```python
from build123d import *

# Parameters (mm, degrees)
SKETCH1_W          = 6.35
SKETCH1_H          = 6.35
EXTRUDE1_DEPTH     = 7.874
SKETCH2_W          = 1.4478
SKETCH2_H          = 1.4478
EXTRUDE2_DEPTH     = 0.635
SKETCH3_W          = 1.016
SKETCH3_H          = 1.016
EXTRUDE3_DEPTH     = 3.937
SKETCH4_R          = 1.693605641
CUT_EXTRUDE1_DEPTH = 0.254
SKETCH5_R          = 0.4826
EXTRUDE4_DEPTH     = 4.826
SKETCH6_W          = 6.35
SKETCH6_H          = 6.35
EXTRUDE5_DEPTH     = 0.9652
SKETCH7_R          = 1.8542
EXTRUDE6_DEPTH     = 6.1468
SKETCH9_R          = 1.236423773
CUT_EXTRUDE2_DEPTH = 5.658092827
SKETCH10_R         = 0.406972167
EXTRUDE7_DEPTH     = 5.658092827
CHAMFER1_SIZE      = 0.508
CHAMFER1_SIZE2     = 0.126658625


with BuildPart() as part:
    # Sketch1 → Extrude1 (new body)
    with BuildSketch(Plane(origin=(0, 0, 0), x_dir=(1, 0, 0), z_dir=(0, 1, 0))):
        with Locations((3.175, 3.175)):
            Rectangle(SKETCH1_W, SKETCH1_H)
    extrude(amount=EXTRUDE1_DEPTH)

    # Sketch2 → Extrude2 (add)
    with BuildSketch(Plane.XZ):
        with Locations((5.6261, -0.7239)):
            Rectangle(SKETCH2_W, SKETCH2_H)
        with Locations((5.6261, -5.6261)):
            Rectangle(SKETCH2_W, SKETCH2_H)
        with Locations((0.7239, -5.6261)):
            Rectangle(SKETCH2_W, SKETCH2_H)
        with Locations((0.7239, -0.7239)):
            Rectangle(SKETCH2_W, SKETCH2_H)
    extrude(amount=EXTRUDE2_DEPTH)

    # Sketch3 → Extrude3 (add)
    with BuildSketch(Plane.XZ.offset(0.635)):
        with Locations((5.715, -0.617649022)):
            Rectangle(SKETCH3_W, SKETCH3_H)
        with Locations((5.715, -5.697649022)):
            Rectangle(SKETCH3_W, SKETCH3_H)
        with Locations((0.635, -5.697649022)):
            Rectangle(SKETCH3_W, SKETCH3_H)
        with Locations((0.635, -0.617649022)):
            Rectangle(SKETCH3_W, SKETCH3_H)
    extrude(amount=EXTRUDE3_DEPTH)

    # Sketch4 → Cut-Extrude1 (cut)
    with BuildSketch(Plane.XZ):
        with Locations(Location((3.175, -3.175, 0), (0, 0, 270))):
            Circle(SKETCH4_R)
    extrude(amount=-CUT_EXTRUDE1_DEPTH, mode=Mode.SUBTRACT)

    # Sketch5 → Extrude4 (add)
    with BuildSketch(Plane.XZ.offset(-0.254)):
        with Locations(Location((3.175, -3.175, 0), (0, 0, 90))):
            Circle(SKETCH5_R)
    extrude(amount=EXTRUDE4_DEPTH)

    # Sketch6 → Extrude5 (add)
    with BuildSketch(Plane.XY):
        with Locations((3.175, 4.699)):
            Rectangle(SKETCH6_W, SKETCH6_H)
    extrude(amount=EXTRUDE5_DEPTH)

    # Sketch7 → Extrude6 (add)
    with BuildSketch(Plane.XY.offset(0.9652)):
        with Locations((3.175, 4.9022)):
            Circle(SKETCH7_R)
    extrude(amount=EXTRUDE6_DEPTH)

    # Sketch8 → Cut-Revolve1 (revolve, cut)
    with BuildSketch(Plane(origin=(0, 4.9022, 0), x_dir=(-1, 0, 0), z_dir=(0, 1, 0))):
        Polygon((-4.767796954, 7.112), (-5.0292, 6.777141647), (-5.0292, 3.959542683), (-4.884349235, 3.83568961), (-4.884349235, 3.47951039), (-5.0292, 3.363076056), (-5.0292, 0.9652), (-5.650551893, 0.9652), (-5.650551893, 7.801111761), align=None)
    revolve(axis=Axis((3.175, 4.9022, 7.112), (0, 0, -1)), mode=Mode.SUBTRACT)

    # Sketch9 → Cut-Extrude2 (cut)
    with BuildSketch(Plane.XY.offset(7.112)):
        with Locations((3.175, 4.9022)):
            Circle(SKETCH9_R)
    extrude(amount=-CUT_EXTRUDE2_DEPTH, mode=Mode.SUBTRACT)

    # Sketch10 → Extrude7 (add)
    with BuildSketch(Plane.XY.offset(1.453907173)):
        with Locations((3.175, 4.9022)):
            Circle(SKETCH10_R)
    extrude(amount=EXTRUDE7_DEPTH)

    # Chamfer1
    chamfer1_edges = [part.edges().sort_by_distance(p)[0] for p in [
        (2.768027833, 4.9022, 7.112),
    ]]
    chamfer1_side = [part.faces().sort_by_distance(p)[0] for p in [
        (2.768027833, 4.9022, 4.282953587),
    ]]
    chamfer(chamfer1_edges, length=CHAMFER1_SIZE, length2=CHAMFER1_SIZE2, reference=chamfer1_side[0])


solid = part.part
```
Work out the finished part from the listing and answer in its coordinate system (mm). A direction names the side the tool comes from. Round coordinates to 2 decimals unless told otherwise and drop trailing zeros. Write each loop counter-clockwise with the first axis right and the second up, starting at its lowest first coordinate (ties: lowest second). Pieces come first, ordered by that corner, then holes. Notation, with made-up numbers: (-15, -30.5) -> (29, -30.5) arc R37 cw to (29, 5.5) -> close; hole circle Ø7 at (18.5, 48). An arc over 180 degrees is marked (long way). Write each question's results on one line, items separated by ' | '.
1) Flat-ended cylindrical pins translate along their axes: pin 1 (1 mm diameter, centred on y = -1.5, z = -1, fed in from -X); pin 2 (0.8 mm diameter, centred on x = 6, y = -2, fed in from +Z); pin 3 (0.6 mm diameter, centred on x = 2, y = 0, fed in from +Z). Find the tip coordinate at first contact, or state that the pin passes through.
Findings:
pin 1: stops at x = 0.13 | pin 2: stops at z = -0.11 | pin 3: stops at z = 0
2) The part is cut by section A-A (z = 5.25). Write down the section's boundary in (x, y) (3 decimals).
Findings:
outline: circle Ø3.708 at (3.175, 4.902); circle Ø0.814 at (3.175, 4.902); hole circle Ø2.473 at (3.175, 4.902)
3) Consider line 1 along Y through (x, z) = (3.25, 6); line 2 along X through (y, z) = (5, 4.5); line 3 along Z through (x, y) = (1, 3.5). Determine where each line is inside the solid, lowest interval first. Write a range as [from, to].
Findings:
line 1: y = [3.05, 3.67], [4.5, 5.3], [6.14, 6.75] | line 2: x = [1.32, 1.94], [2.78, 3.57], [4.41, 5.03] | line 3: z = [-6.35, 0.97]
4) Which of the six approach directions +Z, -Z, +X, -X, +Y, -Y give full straight-line access (tool end or side, diameter ignored) to faces 4 (the flat face through (5.207, -2.6, -0.6)), 5 (the cylindrical face through (2.907, 3.695, 4.323)), 6 (the flat face through (0.6, -2.6, -1.126)), 7 (the cylindrical face through (3.646, -2.125, -3.28)), 8 (the flat face through (0.6, -2.6, -0.11))?
Findings:
face 4: +Z, -Z, -Y | face 5: +Z | face 6: +X, -X, -Y | face 7: -Y | face 8: +Z, +X, -X, -Y
5) The part is cut by section B-B (x = 0.5). Write down the section's boundary in (y, z) (3 decimals).
Findings:
outline: (-4.572, -6.206) -> (-0.635, -6.206) -> (-0.635, -6.35) -> (7.874, -6.35) -> (7.874, 0.965) -> (1.524, 0.965) -> (1.524, 0) -> (-0.635, 0) -> (-0.635, -0.11) -> (-4.572, -0.11) -> (-4.572, -1.126) -> (-0.635, -1.126) -> (-0.635, -1.448) -> (0, -1.448) -> (0, -4.902) -> (-0.635, -4.902) -> (-0.635, -5.19) -> (-4.572, -5.19) -> close
6) The part is cut by section C-C (y = -3). Write down the section's boundary in (x, z) (3 decimals), and give its area (3 significant figures).
Findings:
outline: (0.127, -6.206) -> (1.143, -6.206) -> (1.143, -5.19) -> (0.127, -5.19) -> close; (0.127, -1.126) -> (1.143, -1.126) -> (1.143, -0.11) -> (0.127, -0.11) -> close; circle Ø0.965 at (3.175, -3.175); (5.207, -6.206) -> (6.223, -6.206) -> (6.223, -5.19) -> (5.207, -5.19) -> close; (5.207, -1.126) -> (6.223, -1.126) -> (6.223, -0.11) -> (5.207, -0.11) -> close | area: 4.86 mm²
7) For a pull along X with two mould halves and no side action, classify faces 1 (the flat face through (6, -4.572, -6)), 2 (the cylindrical face through (2.952, 3.207, 3.655)), 3 (the flat face through (5.207, -3, -6)) as +X half, -X half, draft (parallel to the pull), parting line (faces both ways), or undercut.
Findings:
face 1: draft | face 2: parting line | face 3: undercut
8) The part is cut by section D-D (z = -3). Write down the section's boundary in (x, y).
Findings:
outline: (0, 0) -> (1.49, 0) -> (1.49, 0.25) -> (2.73, 0.25) -> (2.73, -4.57) -> (3.62, -4.57) -> (3.62, 0.25) -> (4.86, 0.25) -> (4.86, 0) -> (6.35, 0) -> (6.35, 7.87) -> (0, 7.87) -> close
